For this review, take the finished solid that the model builds, in its own axes (mm). A direction names the side the tool comes from. Give positions to 0.01 mm unless a question says otherwise; leave off trailing zeros. Order: outer loops, then holes, each group sorted by start corner. A loop starts at its lowest first (then second) coordinate and runs counter-clockwise, first axis right, second up.
Item 1: Consider section D-D (z = -60). Give the boundary of the cut face in (x, y).
Item 2: The part is to be moulded in two halves that separate along Z. For faces 5 (the cylindrical face through (102.615, 4.93, 64.249)), 6 (the cylindrical face through (122.15, 5.07, -71.99)), 7 (the flat face through (-1, 60, -1)), 8 (the flat face through (-2, 5, 75)), say which applies: released by +Z, released by -Z, zero draft, split by the parting line, or undercut.
Item 3: For P1, Ø25, axis at x = -24.5, y = 42.5, coming from the +Z side; P2, Ø5, axis at x = -81.5, y = 24, coming from the -Z side; P3, Ø6, axis at y = 35.5, z = 45.5, coming from the +X side, all flat-tipped, find the tip position at first contact; note any pin that passes through.
Item 4: Consider section C-C (y = 54). Give the boundary of the cut face in (x, z).
Item 5: Machinability: for faces 1 (the flat face through (-1, 35, -50)), 2 (the flat face through (100, 35, 1)), 3 (the flat face through (-1, 35, 50)), 4 (the flat face through (-100, 35, 1)), which of the approach directions +Z, -Z, +X, -X, +Y, -Y give a long, thin tool a straight path to every point of the face, cutting with its end or side? Answer none if there is none.
Item 6: For probe 1 along X at (y, z) = (5.5, -65); probe 2 along Z at (x, y) = (-105, 4); probe 3 along Y at (x, z) = (68.5, 55.5), list the stretches that pass through material, from the lowest coordinate up.
Item 7: Consider section B-B (z = 47.5). Give the boundary of the cut face in (x, y).
Item 8: Consider section A-A (x = -105). Give the boundary of the cut face in (y, z).
```python
from build123d import *

# Parameters (mm, degrees)
SKETCH_1_W             = 250
SKETCH_1_H             = 150
EXTRUDE_1_DEPTH        = 10
FILLET_1_R             = 10
SKETCH_2_W             = 200
SKETCH_2_H             = 100
EXTRUDE_2_DEPTH        = 50
HOLE_WIZARD_M6_1_D     = 5
HOLE_WIZARD_M6_1_DEPTH = 15
HOLE_WIZARD_M6_1_TIP   = 1.502151548


with BuildPart() as part:
    # 草图1 → 凸台-拉伸1 (new body)
    with BuildSketch(Plane(origin=(0, 0, 0), x_dir=(1, 0, 0), z_dir=(0, 1, 0))):
        Rectangle(SKETCH_1_W, SKETCH_1_H)
    extrude(amount=EXTRUDE_1_DEPTH)

    # 圆角1
    fillet_1_edges = [part.edges().sort_by_distance(p)[0] for p in [
        (125, 5, 75),
        (-125, 5, 75),
        (-125, 5, -75),
        (125, 5, -75),
    ]]
    fillet(fillet_1_edges, radius=FILLET_1_R)

    # 草图2 → 凸台-拉伸2 (add)
    with BuildSketch(Plane(origin=(0, 10, 0), x_dir=(1, 0, 0), z_dir=(0, 1, 0))):
        Rectangle(SKETCH_2_W, SKETCH_2_H)
    extrude(amount=EXTRUDE_2_DEPTH)

    # M6 螺纹孔1
    with Locations(Plane(origin=(0, 10, 0), x_dir=(1, 0, 0), z_dir=(0, 1, 0))):
        with Locations((-105, -65), (105, 65), (-105, 65), (105, -65)):
            Hole(HOLE_WIZARD_M6_1_D / 2, depth=HOLE_WIZARD_M6_1_DEPTH)
            with Locations((0, 0, -(HOLE_WIZARD_M6_1_DEPTH + HOLE_WIZARD_M6_1_TIP / 2))):  # 118° drill point
                Cone(0, HOLE_WIZARD_M6_1_D / 2, HOLE_WIZARD_M6_1_TIP, mode=Mode.SUBTRACT)


solid = part.part
```
Resolved:
1. outline: (-125, 0) - (125, 0) - (125, 10) - (-125, 10) - close
2. face 5: undercut
2. face 6: released by -Z
2. face 7: zero draft
2. face 8: released by +Z
3. P1: stops at z = 50
3. P2: stops at z = -50
3. P3: stops at x = 100
4. outline: (-100, -50) - (100, -50) - (100, 50) - (-100, 50) - close
5. face 1: -Z, +X, -X, +Y
5. face 2: +Z, -Z, +X, +Y
5. face 3: +Z, +X, -X, +Y
5. face 4: +Z, -Z, -X, +Y
6. probe 1: x = -125 to -107.5, -102.5 to 102.5, 107.5 to 125
6. probe 2: z = -75 to -67.5, -62.5 to 62.5, 67.5 to 75
6. probe 3: y = 0 to 10
7. outline: (-125, 0) - (125, 0) - (125, 10) - (100, 10) - (100, 60) - (-100, 60) - (-100, 10) - (-125, 10) - close
8. outline: (0, -75) - (10, -75) - (10, -67.5) - (0, -67.5) - close; (0, -62.5) - (10, -62.5) - (10, 62.5) - (0, 62.5) - close; (0, 67.5) - (10, 67.5) - (10, 75) - (0, 75) - close
